from build123d import *

# Parameters (mm, degrees)
F0_R     = 4.25
F1_DEPTH = 7
F3_DEPTH = 25
F4_R     = 4
F5_DEPTH = 25


with BuildPart() as f1:
    # F0 (on Top) → F1 (new body)
    with BuildSketch(Plane.XY):
        with BuildLine():
            Line((2, 5.5), (-26, 5.5))
            ThreePointArc((-26, 5.5), (-28.828427, 4.328427), (-30, 1.5))
            Line((-30, 1.5), (-30, -1.5))
            ThreePointArc((-30, -1.5), (-28.828427, -4.328427), (-26, -5.5))
            Line((-26, -5.5), (2, -5.5))
            ThreePointArc((2, -5.5), (4.828427, -4.328427), (6, -1.5))
            Line((6, -1.5), (6, 1.5))
            ThreePointArc((6, 1.5), (4.828427, 4.328427), (2, 5.5))
        make_face()
        Circle(F0_R, mode=Mode.SUBTRACT)
    extrude(amount=F1_DEPTH)

    # F2 (on face) → F3 (cut)
    with BuildSketch(Plane.XZ.offset(5.5)):
        with BuildLine():
            Line((-16.256757, 0), (-9, 0))
            ThreePointArc((-9, 0), (-12.628379, 2.037), (-16.256757, 0))
        make_face()
    extrude(amount=-F3_DEPTH, mode=Mode.SUBTRACT)

    # F4 (on face) → F5 (cut)
    with BuildSketch(Plane.XY.offset(7)):
        with Locations((-25, 0)):
            Circle(F4_R)
    extrude(amount=-F5_DEPTH, mode=Mode.SUBTRACT)


solid = f1.part
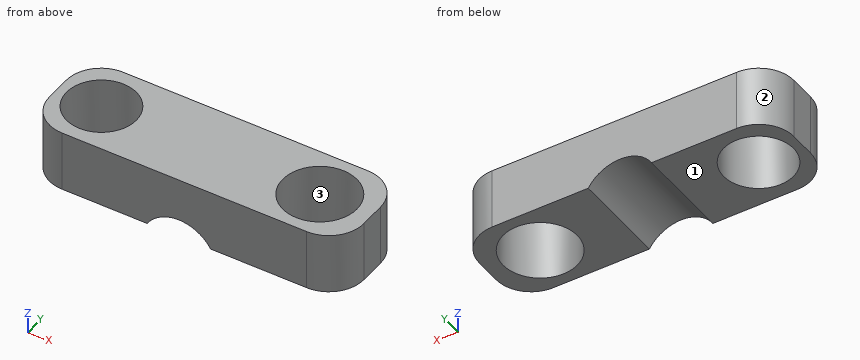
Can you work these out from the model? Positions are in its coordinate system, mm. Face numbers are marked on the shaded views. Give positions to 0.01 mm unless a question says otherwise; leave off trailing zeros. Loops run counter-clockwise (first coordinate to the right, second up) from the corner with the lowest first, then second, coordinate; pieces in that order, holes last. Notation, with made-up numbers: (-19, 6.5) - (-1, 6.5) arc R31 cw to (-1, 30.5) - close; hole circle Ø7 at (57, 37). An arc over 180 degrees is marked (long way). One line per item, written item: value.
(1) If we section it at D-D, the plane x = -25: List the corners of the cut face in (y, z) for me.
Verdict:
outline: (-5.5, 0) - (-4, 0) - (-4, 7) - (-5.5, 7) - close; (4, 0) - (5.5, 0) - (5.5, 7) - (4, 7) - close
(2) If we section it at A-A, the plane x = 0: List the corners of the cut face in (y, z) for me, plus the area to 3 significant figures.
Verdict:
outline: (-5.5, 0) - (-4.25, 0) - (-4.25, 7) - (-5.5, 7) - close; (4.25, 0) - (5.5, 0) - (5.5, 7) - (4.25, 7) - close
area: 17.5 mm^2
(3) If we mould it in two halves opening along X, with no side actions, what happens to the marked faces 1, 2 and 3? For each: released by +X, released by -X, zero draft, split by the parting line, or undercut.
Verdict:
face 1: zero draft
face 2: released by -X
face 3: undercut
(4) I'm going to push flat-ended pins straight in: pin 1 (5 mm diameter, centred on x = 0, y = 0, fed in from -Z); pin 2 (1.5 mm diameter, centred on y = -3.5, z = 5, fed in from -X); pin 3 (4 mm diameter, centred on x = -11.5, z = 1, fed in from +Y); pin 4 (1 mm diameter, centred on y = -3, z = 4.5, fed in from -X). Where does each tip first touch, or does it pass through?
Verdict:
pin 1: through
pin 2: x = -29.8
pin 3: y = 5.5
pin 4: x = -29.87
(5) If we section it at B-B, the plane z = 1.25: List the corners of the cut face in (x, y) for me.
Verdict:
outline: (-30, -1.5) arc R4 ccw to (-26, -5.5) - (-15.09, -5.5) - (-15.09, 5.5) - (-26, 5.5) arc R4 ccw to (-30, 1.5) - close; (-10.16, -5.5) - (2, -5.5) arc R4 ccw to (6, -1.5) - (6, 1.5) arc R4 ccw to (2, 5.5) - (-10.16, 5.5) - close; hole circle Ø8 at (-25, 0); hole circle Ø8.5 at (0, 0)
(6) I need wall thicknesses on line 1 along Y through (x, z) = (-25, 1); line 2 along X through (y, z) = (1.75, 5.5); line 3 along X through (y, z) = (-2, 1.25). Which ranges of each line are inside material? Lowest first, please.
Verdict:
line 1: -5.5 to -4, 4 to 5.5
line 2: -29.99 to -28.6, -21.4 to -3.87, 3.87 to 5.99
line 3: -29.97 to -28.46, -21.54 to -15.09, -10.16 to -3.75, 3.75 to 5.97
(7) If we section it at C-C, the plane y = 0: List the corners of the cut face in (x, z) for me.
Verdict:
outline: (-30, 0) - (-29, 0) - (-29, 7) - (-30, 7) - close; (-21, 0) - (-16.26, 0) arc R4.25 cw to (-9, 0) - (-4.25, 0) - (-4.25, 7) - (-21, 7) - close; (4.25, 0) - (6, 0) - (6, 7) - (4.25, 7) - close
